Verification items for the finished model (mm, model axes). A direction names the side the tool comes from. Coordinates: 2 decimals unless noted, no trailing zeros. Write each loop counter-clockwise with the first axis right and the second up, starting at its lowest first coordinate (ties: lowest second). Pieces come first, ordered by that corner, then holes. Notation, with made-up numbers: (60.5, 51.25) -> (65.5, 51.25) arc R15 cw to (65.5, 74.25) -> close; hole circle Ø11 at (-37, -31). An arc over 180 degrees is marked (long way). Answer in a Markdown table with one row per item.
```python
from build123d import *

# Parameters (mm, degrees)
SKETCH_1_R          = 42.5
EXTRUDE_1_DEPTH     = 20
SKETCH_2_R          = 37.5
EXTRUDE_2_DEPTH     = 30
SKETCH_3_R          = 24
EXTRUDE_3_DEPTH     = 89
SKETCH_5_R          = 20
EXTRUDE_4_DEPTH     = 4.5
SKETCH_7_W          = 15
SKETCH_7_H          = 4.5
EXTRUDE_5_DEPTH     = 10
SKETCH_8_W          = 4.5
SKETCH_8_H          = 15
EXTRUDE_6_DEPTH     = 10
SKETCH_9_W          = 4.5
SKETCH_9_H          = 15
EXTRUDE_7_DEPTH     = 10
EXTRUDE_8_DEPTH     = 15
EXTRUDE_9_DEPTH     = 15
EXTRUDE_10_DEPTH    = 15
SKETCH_13_R         = 1
CUT_EXTRUDE_1_DEPTH = 51
SKETCH_14_R         = 1
CUT_EXTRUDE_2_DEPTH = 62.225952642
SKETCH_15_R         = 1
CUT_EXTRUDE_3_DEPTH = 70.88620668
SKETCH_18_W         = 4.5
SKETCH_18_H         = 10
CUT_EXTRUDE_4_DEPTH = 3.25
SKETCH_19_W         = 4.5
SKETCH_19_H         = 10
CUT_EXTRUDE_5_DEPTH = 3.25
SKETCH_20_W         = 10
SKETCH_20_H         = 4.5
CUT_EXTRUDE_6_DEPTH = 3.25


with BuildPart() as part:
    # ｽｹｯﾁ1 → ﾎﾞｽ - 押し出し1 (new body)
    with BuildSketch(Plane.XY):
        Circle(SKETCH_1_R)
    extrude(amount=EXTRUDE_1_DEPTH)

    # ｽｹｯﾁ2 → ﾎﾞｽ - 押し出し2 (add)
    with BuildSketch(Plane.XY.offset(20)):
        Circle(SKETCH_2_R)
    extrude(amount=EXTRUDE_2_DEPTH)

    # ｽｹｯﾁ3 → ﾎﾞｽ - 押し出し3 (add)
    with BuildSketch(Plane.XY.offset(50)):
        with Locations((0, 5)):
            Circle(SKETCH_3_R)
    extrude(amount=EXTRUDE_3_DEPTH)

    # ｽｹｯﾁ5 → ﾎﾞｽ - 押し出し4 (add)
    with BuildSketch(Plane.XY.offset(139)):
        with Locations((0, 5)):
            Circle(SKETCH_5_R)
    extrude(amount=EXTRUDE_4_DEPTH)

    # ｽｹｯﾁ7 → ﾎﾞｽ - 押し出し5 (add)
    with BuildSketch(Plane(origin=(0, 25, 0), x_dir=(1, 0, 0), z_dir=(0, 1, 0))):
        with Locations((0, -141.25)):
            Rectangle(SKETCH_7_W, SKETCH_7_H)
    extrude(amount=-EXTRUDE_5_DEPTH)

    # ｽｹｯﾁ8 → ﾎﾞｽ - 押し出し6 (add)
    with BuildSketch(Plane(origin=(-15.155444566, -8.75, 0), x_dir=(0, 0, 1), z_dir=(-0.866025404, -0.5, 0))):
        with Locations((141.25, 4.330127019)):
            Rectangle(SKETCH_8_W, SKETCH_8_H)
    extrude(amount=-EXTRUDE_6_DEPTH)

    # ｽｹｯﾁ9 → ﾎﾞｽ - 押し出し7 (add)
    with BuildSketch(Plane(origin=(15.155444566, -8.75, 0), x_dir=(0, 0, -1), z_dir=(0.866025404, -0.5, 0))):
        with Locations((-141.25, 4.330127019)):
            Rectangle(SKETCH_9_W, SKETCH_9_H)
    extrude(amount=-EXTRUDE_7_DEPTH)

    # ｽｹｯﾁ10 → ﾎﾞｽ - 押し出し8 (add)
    with BuildSketch(Plane(origin=(5.915063509, 10.245190528, 0), x_dir=(0.866025404, -0.5, 0), z_dir=(0.5, 0.866025404, 0))):
        with BuildLine():
            Line((17.5, -143.5), (18.5, -143.5))
            ThreePointArc((18.5, -143.5), (20.75, -141.25), (18.5, -139))
            Line((18.5, -139), (17.5, -139))
            Line((17.5, -139), (17.5, -143.5))
        make_face()
    extrude(amount=-EXTRUDE_8_DEPTH)

    # ｽｹｯﾁ11 → ﾎﾞｽ - 押し出し9 (add)
    with BuildSketch(Plane.ZY.offset(7.5)):
        with BuildLine():
            Line((139, 25), (143.5, 25))
            Line((143.5, 25), (143.5, 26))
            ThreePointArc((143.5, 26), (141.25, 28.25), (139, 26))
            Line((139, 26), (139, 25))
        make_face()
    extrude(amount=-EXTRUDE_9_DEPTH)

    # ｽｹｯﾁ12 → ﾎﾞｽ - 押し出し10 (add)
    with BuildSketch(Plane(origin=(1.584936491, -2.745190528, 0), x_dir=(0.866025404, 0.5, 0), z_dir=(0.5, -0.866025404, 0))):
        with BuildLine():
            Line((-17.5, 139), (-17.5, 143.5))
            Line((-17.5, 143.5), (-18.5, 143.5))
            ThreePointArc((-18.5, 143.5), (-20.75, 141.25), (-18.5, 139))
            Line((-18.5, 139), (-17.5, 139))
        make_face()
    extrude(amount=-EXTRUDE_10_DEPTH)

    # ｽｹｯﾁ13 → ｶｯﾄ - 押し出し1 (cut, through all)
    with BuildSketch(Plane.ZY.offset(7.5)):
        with Locations((141.25, 26)):
            Circle(SKETCH_13_R)
    extrude(amount=-CUT_EXTRUDE_1_DEPTH, mode=Mode.SUBTRACT)

    # ｽｹｯﾁ14 → ｶｯﾄ - 押し出し2 (cut, through all)
    with BuildSketch(Plane(origin=(1.584936491, -2.745190528, 0), x_dir=(-0.866025404, -0.5, 0), z_dir=(0.5, -0.866025404, 0))):
        with Locations((18.5, -141.25)):
            Circle(SKETCH_14_R)
    extrude(amount=-CUT_EXTRUDE_2_DEPTH, mode=Mode.SUBTRACT)

    # ｽｹｯﾁ15 → ｶｯﾄ - 押し出し3 (cut, through all)
    with BuildSketch(Plane(origin=(5.915063509, 10.245190528, 0), x_dir=(0.866025404, -0.5, 0), z_dir=(0.5, 0.866025404, 0))):
        with Locations((18.5, -141.25)):
            Circle(SKETCH_15_R)
    extrude(amount=-CUT_EXTRUDE_3_DEPTH, mode=Mode.SUBTRACT)

    # ｽｹｯﾁ18 → ｶｯﾄ - 押し出し4 (cut)
    with BuildSketch(Plane(origin=(-17.970027129, -10.375, 0), x_dir=(0, 0, 1), z_dir=(-0.866025404, -0.5, 0))):
        with Locations((141.25, 4.330127019)):
            Rectangle(SKETCH_18_W, SKETCH_18_H)
    extrude(amount=-CUT_EXTRUDE_4_DEPTH, mode=Mode.SUBTRACT)

    # ｽｹｯﾁ19 → ｶｯﾄ - 押し出し5 (cut)
    with BuildSketch(Plane(origin=(17.970027129, -10.375, 0), x_dir=(0, 0, -1), z_dir=(0.866025404, -0.5, 0))):
        with Locations((-141.25, 4.330127019)):
            Rectangle(SKETCH_19_W, SKETCH_19_H)
    extrude(amount=-CUT_EXTRUDE_5_DEPTH, mode=Mode.SUBTRACT)

    # ｽｹｯﾁ20 → ｶｯﾄ - 押し出し6 (cut)
    with BuildSketch(Plane(origin=(0, 28.25, 0), x_dir=(1, 0, 0), z_dir=(0, 1, 0))):
        with Locations((0, -141.25)):
            Rectangle(SKETCH_20_W, SKETCH_20_H)
    extrude(amount=-CUT_EXTRUDE_6_DEPTH, mode=Mode.SUBTRACT)


solid = part.part
```
1. Sectioned sample at D-D, the plane x = -36. Record the cut outline in (y, z).
Findings below:
| item | result |
|---|---|
| outline | (-22.59, 0) -> (22.59, 0) -> (22.59, 20) -> (10.5, 20) -> (10.5, 50) -> (-10.5, 50) -> (-10.5, 20) -> (-22.59, 20) -> close |
2. Sectioned sample at C-C, the plane z = 88. Record the cut outline in (x, y).
Findings below:
| item | result |
|---|---|
| outline | circle Ø48 at (0, 5) |
3. Sectioned sample at A-A, the plane x = 0. Record the cut outline in (y, z).
Findings below:
| item | result |
|---|---|
| outline | (-42.5, 0) -> (42.5, 0) -> (42.5, 20) -> (37.5, 20) -> (37.5, 50) -> (29, 50) -> (29, 139) -> (25, 139) -> (25, 143.5) -> (-15, 143.5) -> (-15, 139) -> (-19, 139) -> (-19, 50) -> (-37.5, 50) -> (-37.5, 20) -> (-42.5, 20) -> close |
4. Go/stop test with flat-tipped pins: pin 1 (3.5 mm diameter, centred on x = 1.5, z = 141.5, fed in from +Y); pin 2 (1.5 mm diameter, centred on y = 27, z = 37, fed in from -X); pin 3 (1 mm diameter, centred on x = 21, z = 38.5, fed in from -Y). Record where each tip stops, or that it passes through.
Findings below:
| item | result |
|---|---|
| pin 1 | stops at y = 25 |
| pin 2 | stops at x = -26.78 |
| pin 3 | stops at y = -31.4 |
5. Access from +Z, -Z, +X, -X, +Y, -Y to the whole of each face (thin tool, end or side, straight path). Record for faces 5 (the face through (-16.873, -10.515, 141.218)), 6 (the face through (0, 25, 141)), 7 (the face through (16.873, -10.515, 141.282)), 8 (the face through (-33.727, -25.861, 9.86)), 9 (the face through (-13.468, -11.436, 140.782)).
Findings below:
| item | result |
|---|---|
| face 5 | +Z, -X |
| face 6 | +Z, +Y |
| face 7 | +Z, +X |
| face 8 | +Z, -Z |
| face 9 | +Z, -Y |
6. Material ranges on probe 1 along Z at (x, y) = (8, 38); probe 2 along Y at (x, z) = (-6, 141); probe 3 along Z at (x, y) = (16.5, 16.5), recorded low to high. Write a range as from..to.
Findings below:
| item | result |
|---|---|
| probe 1 | z = 0..20 |
| probe 2 | y = -14.08..25.03, 26.97..28.24 |
| probe 3 | z = 0..139 |
7. Release check for a two-part mould opening along X. For faces 1 (the face through (0, -15, 141)), 2 (the face through (-20.968, 1.554, 140.782)), 3 (the face through (-5, 27, 142)), 4 (the face through (17.41, 14.84, 141.22)) record: released by +X, released by -X, zero draft, split by the parting line, or undercut.
Findings below:
| item | result |
|---|---|
| face 1 | undercut |
| face 2 | released by -X |
| face 3 | undercut |
| face 4 | released by +X |
8. Sectioned sample at B-B, the plane y = 5. Record the cut outline in (x, z), and give its area (3 significant figures).
Findings below:
| item | result |
|---|---|
| outline | (-42.2, 0) -> (42.2, 0) -> (42.2, 20) -> (37.17, 20) -> (37.17, 50) -> (24, 50) -> (24, 139) -> (20, 139) -> (20, 143.5) -> (-20, 143.5) -> (-20, 139) -> (-24, 139) -> (-24, 50) -> (-37.17, 50) -> (-37.17, 20) -> (-42.2, 20) -> close |
| area | 8,370 mm² |
